Design review of the part built by this model. Coordinates are the model's own, in mm. A direction names the side the tool comes from. Round coordinates to 2 decimals unless told otherwise and drop trailing zeros. Loops run counter-clockwise (first coordinate to the right, second up) from the corner with the lowest first, then second, coordinate; pieces in that order, holes last. Notation, with made-up numbers: (-38.5, 86.25) - (11.5, 86.25) arc R19 ccw to (11.5, 116.25) - close; hole circle Ø4 at (60, 81.5). An arc over 180 degrees is marked (long way). Answer as CSV lines item,"result". Start each with the question number.
(1) For P1, Ø6, axis at y = 593, z = 55.5, coming from the -X side; P2, Ø1, axis at y = 226.5, z = 52, coming from the +X side, all flat-tipped, find the tip position at first contact; note any pin that passes through.
(2) Consider section B-B (y = 436.5). Give the boundary of the cut face in (x, z).
(3) Wall thickness on L1, parallel to Y at x = 658, z = 322; L2, parallel to Z at x = 697, y = 439.5; L3, parallel to Y at x = 1120.5, z = 161.5: over which ranges is each line inside the solid? List them lowest first.
(4) Consider section C-C (y = 726). Give the boundary of the cut face in (x, z), and give its area (3 significant figures).
(5) Consider section A-A (x = 1837.5). Give the boundary of the cut face in (y, z), and give its area (3 significant figures).
(6) For faces 5 (the flat face through (857, 425, 737.552)), 6 (the flat face through (1722, 736, 534.352)), 7 (the flat face through (1722, 123, 127.952)), list the 3-axis set-ups (+Z, -Z, +X, -X, +Y, -Y) from which the entire face can be reached by the end or side of a thin tool; tool diameter is ignored.
(7) Mouldability with a two-part tool opening along Y and no side actions: class faces 1 (the flat face through (1052, -75.582, 325)), 2 (the flat face through (1052, 940.418, 325)), 3 (the flat face through (2133.6, 78, 334)), 4 (the cylindrical face through (1051.85, 650.46, 399.82)) as released by +Y, released by -Y, zero draft, split by the parting line, or undercut.
(8) Consider section D-D (x = 1054). Give the boundary of the cut face in (y, z).
from build123d import *
from build123d import SkipClean  # not in build123d's __all__

# Parameters (mm, degrees)
F0_W     = 1016
F0_H     = 812.8
F0_R     = 228.6
F1_DEPTH = 2133.6
F2_W     = 812.8
F2_H     = 203.2
F3_DEPTH = 1016.001


with BuildPart() as f1:
    # F0 (on Right) → F1 (new body)
    with BuildSketch(Plane.YZ):
        with Locations((432.4176223874, 331.1518777847)):
            Rectangle(F0_W, F0_H)
        with Locations((432.4176223874, 331.1518777847)):
            Circle(F0_R, mode=Mode.SUBTRACT)
    extrude(amount=F1_DEPTH)

    # F2 (on face) → F3 (cut, through all)
    with BuildSketch(Plane.XZ.offset(75.5823776126)):
        with BuildLine():
            Line((0, 737.5518777847), (0, 331.1518777847))
            ThreePointArc((0, 331.1518777847), (119.0318041258, 618.5200736589), (406.4, 737.5518777847))
            Line((406.4, 737.5518777847), (0, 737.5518777847))
        make_face()
        with BuildLine():
            Line((0, 331.1518777847), (0, -75.2481222153))
            Line((0, -75.2481222153), (406.4, -75.2481222153))
            ThreePointArc((406.4, -75.2481222153), (119.0318041258, 43.7836819105), (0, 331.1518777847))
        make_face()
        with Locations((1727.2, 26.3518777847)):
            Rectangle(F2_W, F2_H)
        with Locations((1727.2, 635.9518777847)):
            Rectangle(F2_W, F2_H)
    with SkipClean():  # cleaning this boolean's faces spoils the solid; the shape is the same uncleaned
        extrude(amount=-F3_DEPTH, mode=Mode.SUBTRACT)


solid = f1.part
Determined:
1,P1,"stops at x = 105.03"
1,P2,"stops at x = 1320.8"
2,outline,"(70.36, 102.59) arc R406.4 ccw to (406.4, -75.25) - (1320.8, -75.25) - (1320.8, 102.59) - close; (70.36, 559.72) - (1320.8, 559.72) - (1320.8, 737.55) - (406.4, 737.55) arc R406.4 ccw to start"
3,L1,"y = -75.58 to 204, 660.83 to 940.42"
3,L2,"z = -75.25 to 102.66, 559.64 to 737.55"
3,L3,"y = -75.58 to 279.2, 585.64 to 940.42"
4,outline,"(406.4, -75.25) - (1320.8, -75.25) - (1320.8, 127.95) - (2133.6, 127.95) - (2133.6, 534.35) - (1320.8, 534.35) - (1320.8, 737.55) - (406.4, 737.55) arc R406.4 ccw to start"
4,area,"1,330,000 mm^2"
5,outline,"(-75.58, 127.95) - (327.69, 127.95) arc R228.6 cw to (327.69, 534.35) - (-75.58, 534.35) - close; (537.14, 127.95) - (940.42, 127.95) - (940.42, 534.35) - (537.14, 534.35) arc R228.6 cw to start"
5,area,"256,000 mm^2"
6,face 5,"+Z, +X, -X, +Y, -Y"
6,face 6,"+Z, +X, +Y, -Y"
6,face 7,"-Z, +X, +Y, -Y"
7,face 1,"released by -Y"
7,face 2,"released by +Y"
7,face 3,"zero draft"
7,face 4,"undercut"
8,outline,"(-75.58, -75.25) - (940.42, -75.25) - (940.42, 737.55) - (-75.58, 737.55) - close; hole circle Ø457.2 at (432.42, 331.15)"
